The model under review builds one solid part; all positions refer to its coordinate system, in mm. A direction names the side the tool comes from. Round coordinates to 2 decimals unless told otherwise and drop trailing zeros. Write each loop counter-clockwise with the first axis right and the second up, starting at its lowest first coordinate (ties: lowest second). Pieces come first, ordered by that corner, then holes.
Item 1: Machinability: for faces 4 (the face through (-24, 38, -35)), 5 (the face through (0, 19.5, -20)), 6 (the face through (-1, 24, -80.533)), 7 (the face through (0, 22, -9.757)), which of the approach directions +Z, -Z, +X, -X, +Y, -Y give a long, thin tool a straight path to every point of the face, cutting with its end or side? Answer none if there is none.
Item 2: Add section C-C (x = 23). Give the boundary of the cut face in (y, z), plus the area to 3 significant figures.
Item 3: Add section A-A (x = -6). Give the boundary of the cut face in (y, z), plus the area to 3 significant figures.
Item 4: Draft analysis for pull direction X (two halves, no side actions). For faces 1 (the face through (23, 28, -40)), 2 (the face through (30.5, 22, -20)), 3 (the face through (0, 80, -1)), state which applies: +X half, -X half, draft (parallel to the pull), parting line (faces both ways), or undercut.
Item 5: Clearance check with flat-ended pins moving along their axes: pin 1 Ø6 at (x, y) = (-13, 41) entering from -Z; pin 2 Ø2 at (x, y) = (44, 75) entering from -Z; pin 3 Ø5 at (x, z) = (14.5, -61.5) entering from -Y; pin 4 Ø2 at (x, z) = (-25.5, -59) entering from +Y. State where each tip first meets the part, or that it passes through.
Item 6: To check wall thickness, follow L1, parallel to Z at x = -35, y = 19; L2, parallel to X at y = 59, z = -43.5; L3, parallel to Z at x = 2.5, y = 10. State the ranges of each line that lie inside material, in increasing order.
Item 7: Add section B-B (y = 11.5). Give the boundary of the cut face in (x, z), plus the area to 3 significant figures.
Item 8: Add section D-D (z = -44.5). Give the boundary of the cut face in (x, y), plus the area to 3 significant figures.
Autodesk Inventor part; units mm, degrees
ref_plane "YZ Plane" through (0, 0, 0) normal (1, 0, 0) x (0, 1, 0)
ref_plane "XZ Plane" through (0, 0, 0) normal (0, 1, 0) x (-1, 0, 0)
ref_plane "XY Plane" through (0, 0, 0) normal (0, 0, 1) x (1, 0, 0)
sketch "Esboço1" plane through (0, 0, 0) normal (1, 0, 0) x (0, 1, 0)
  line L0 (0, 0) -> (80, 0)
  line L1 (80, 0) -> (80, -52)
  line L2 (80, -97) -> (0, -97)
  line L3 (0, -97) -> (0, 0)
  line L4 (80, 0) -> (0, 0)
  line L5 (0, 0) -> (0, -60)
  line L6 (80, -60) -> (80, 0)
  line L7 (0, 0) -> (0, -19.5)
  line L8 (19.5, 0) -> (0, 0)
  line L9 (0, -98) -> (0, -97)
  line L10 (0, -97) -> (40, -97)
  line L11 (0, 0) -> (0, -20)
  line L12 (80, 0) -> (80, -52)
  line L13 (80, -52) -> (0, -52)
  line L14 (0, -52) -> (0, -97)
  line L15 (0, -97) -> (80, -97)
  line L16 (80, -97) -> (80, -52)
  line L17 (0, -74.5) -> (0, -97)
  line L18 (0, -97) -> (80, -97)
  line L19 (80, -97) -> (80, -74.5)
  line L20 (80, -52) -> (80, -78.5)
  line L21 (53.5, -78.5) -> (28.1691, -78.5)
  line L22 (80, -52) -> (53.5, -78.5)
  arc A0 (0.0257, -97) -> (0, -98) centre (19.5, -98) ccw
  line L23 (80, -52) -> (80, -54)
  line L24 (80, -54) -> (53.5, -80.533)
  line L25 (53.5, -80.533) -> (28.1691, -80.533)
  line L26 (28.1691, -80.533) -> (28.1691, -78.5)
  arc A1 (18.9926, -80.533) -> (0, -98) centre (23.5809, -104.5813) ccw
  line L27 (28.1691, -80.533) -> (18.9926, -80.533)
  circle A2 centre (20, -20) radius 18.5
  line L28 (20, -38.5) -> (0, -38.5)
  line L29 (20, -1.5) -> (0, -1.5)
  point P0 (0, -78.5)
  point P1 (80, -78.5)
  point P2 (0.3022, -97)
  dimension "d0" = 80
  dimension "d1" = 97
  dimension "d6" = 20
  dimension "d13" = 52
  dimension "d14" = 26.5
  dimension "d15" = 26.5
  dimension "d16" = 26.5
  dimension "d17" = 19.5
  dimension "d19" = 2
  dimension "d20" = 37.5
  dimension "d75" = 37
sketch "Esboço2" plane through (0, 0, 0) normal (1, 0, 0) x (0, 1, 0)
  point P0 (0, 0)
extrude "Extrusão1" add sketch "Esboço1" along normal mid plane 97 contours L0 L1 L13 L3 L28 A2 L29 | L29 A2 L28 L3 | A2 | L22 L21 L26 L27 A1 L2 L3 L13 | L2 A0 L9 | A1 A0 L2
sketch "Esboço3" plane through (0, 0, 0) normal (1, 0, 0) x (0, 1, 0)
  line L0 (0, 0) -> (80, 0)
  line L1 (80, 0) -> (80, -2.5)
  line L2 (80, 0) -> (80, -52)
  line L3 (80, -2.5) -> (80, -5)
  line L4 (80, -2.5) -> (77, -2.5)
  line L5 (53.5, -78.5) -> (28.1691, -78.5)
  line L6 (77, -2.5) -> (42, -2.5)
  line L7 (42, -2.5) -> (42, -78.5)
  line L8 (42, -78.5) -> (77, -78.5)
  line L9 (77, -78.5) -> (77, -2.5)
  line L10 (28.1691, -78.5) -> (31.1691, -78.5)
  line L11 (28.1691, -78.5) -> (42, -78.5)
  line L12 (42, -78.5) -> (42, -40.5)
  line L13 (28.1691, -78.5) -> (42, -78.5)
  line L14 (42, -78.5) -> (42, -42.2949)
  line L15 (42, -42.2949) -> (28.1691, -42.2949)
  line L16 (28.1691, -42.2949) -> (28.1691, -78.5)
  line L17 (28.1691, -42.2949) -> (4.792, -42.2949)
  line L18 (4.792, -42.2949) -> (4.792, -71.2859)
  line L19 (4.792, -71.2859) -> (28.1691, -71.2859)
  point P0 (20, 0)
  dimension "d27" = 2.5
  dimension "d28" = 2.5
  dimension "d29" = 3
  dimension "d30" = 35
extrude "Extrusão2" cut sketch "Esboço3" along normal mid plane 91
sketch "Esboço4" plane through (-48.5, 80, 0) normal (0, 1, 0) x (1, 0, 0)
  line L0 (0, 0) -> (0, 52)
  line L1 (0, 0) -> (97, 0)
  line L2 (3, 2.5) -> (3, 55)
  line L3 (94, 2.5) -> (3, 2.5)
  line L4 (3, 2.5) -> (93.6926, 2.5)
  line L5 (93.6926, 2.5) -> (93.6926, 52)
  line L6 (93.6926, 52) -> (3, 52)
  line L7 (3, 52) -> (3, 2.5)
  point P0 (48.5, 0)
extrude "Extrusão3" cut sketch "Esboço4" against normal blind 8.5
sketch "Esboço5" plane through (-45.5, 77, -52) normal (0, 0, 1) x (1, 0, 0)
  line L0 (91, 0) -> (0, 0)
  line L1 (0, 0) -> (4, 0)
  line L2 (4, 0) -> (4, -4)
  line L3 (4, -4) -> (0, -4)
  line L4 (0, -4) -> (0, 0)
  line L5 (91, -23.5) -> (91, 0)
  line L6 (91, 0) -> (87, 0)
  line L7 (87, 0) -> (87, -4)
  line L8 (87, -4) -> (91, -4)
  line L9 (91, -4) -> (91, 0)
  line L10 (0, 3) -> (0, 0)
  line L11 (0, 3) -> (4, 3)
  line L12 (4, 3) -> (4, 0)
  line L13 (4, 0) -> (0, 0)
  line L14 (0, 0) -> (0, 3)
  line L15 (87, 3) -> (91, 3)
  line L16 (91, 3) -> (91, 0)
  line L17 (91, 0) -> (87, 0)
  line L18 (87, 0) -> (87, 3)
  point P0 (45.5, -77)
  point P1 (91, -4)
  dimension "d38" = 4
  dimension "d39" = 4
  dimension "d40" = 4
extrude "Extrusão4" add sketch "Esboço5" along normal blind 49.5
sketch "Esboço6" plane through (45.5, 4.792, -42.2949) normal (0, 0, -1) x (-1, 0, 0)
  line L0 (0, 37.208) -> (0, 33.208)
  line L1 (17, 33.208) -> (27, 33.208)
  line L2 (27, 33.208) -> (27, 23.208)
  line L3 (27, 23.208) -> (17, 23.208)
  line L4 (17, 23.208) -> (17, 33.208)
  line L5 (0, 37.208) -> (91, 37.208)
  line L6 (91, 37.208) -> (87, 37.208)
  line L7 (-3, 35.208) -> (94, 35.208)
  line L8 (91, 37.208) -> (91, 33.208)
  line L9 (74, 33.208) -> (64, 33.208)
  line L10 (64, 33.208) -> (64, 23.208)
  line L11 (64, 23.208) -> (74, 23.208)
  line L12 (74, 23.208) -> (74, 33.208)
  line L13 (91, 33.208) -> (74, 33.208)
  point P0 (45.5, -4.792)
  dimension "d43" = 4
  dimension "d44" = 17
  dimension "d45" = 10
  dimension "d46" = 10
  dimension "d52" = 10
  dimension "d53" = 10
  dimension "d54" = 17
extrude "Extrusão5" cut sketch "Esboço6" against normal blind 14 contours L12 L11 L10 L9 | L1 L2 L3 L4
sketch "Esboço9" plane through (48.5, 0, 0) normal (1, 0, 0) x (0, 0, -1)
  circle A0 centre (20, 20) radius 18.5
  line L0 (1.5, 20) -> (1.5, 0)
  line L1 (98, 0) -> (0, 0)
  line L2 (38.5, 20) -> (38.5, 0)
  line L3 (20, 24) -> (1.9376, 24)
  line L4 (20, 24) -> (38.0624, 24)
  line L5 (20, 19.5) -> (38.5, 19.5)
  line L6 (20, 19.5) -> (1.5, 19.5)
  point P0 (38.5, 0)
  point P1 (1.5068, 19.5)
  point P2 (38.4932, 19.5)
  dimension "d76" = 37
  dimension "d81" = 4.5
extrude "Extrusão7" cut sketch "Esboço9" against normal blind 97
extrude "Extrusão8" add sketch "Esboço9" against normal blind 97 contours A0 L5 L6 L3 L4
sketch "Esboço10" plane through (48.5, 19.5, -38.4932) normal (0, -1, 0) x (1, 0, 0)
  line L0 (-97, 0) -> (-97, 36.9865)
  line L1 (0, -13.5068) -> (0, 38.4932)
  line L2 (0, 0.4309) -> (0, 36.5556)
  line L3 (0, -0.0068) -> (-97, -0.0068)
  line L4 (-97, 36.9865) -> (-79, 36.9865)
  line L5 (-79, 36.9865) -> (-79, -0.0068)
  line L6 (-79, -0.0068) -> (-97, -0.0068)
  line L7 (-97, -0.0068) -> (-97, 36.9865)
  line L8 (0, 36.9865) -> (-97, 36.9865)
  line L9 (-18, 36.9865) -> (0, 36.9865)
  line L10 (0, 36.9865) -> (0, -0.0068)
  line L11 (0, -0.0068) -> (-18, -0.0068)
  line L12 (-18, -0.0068) -> (-18, 36.9865)
  point P0 (-48.5, 38.4932)
extrude "Extrusão9" cut sketch "Esboço10" against normal blind 4.5 contours L0 L4 L5 L3 L7 | L8 L1 L3 L12
sketch "Esboço11" plane through (-30.5, 19.5, -1.5068) normal (0, -1, 0) x (1, 0, 0)
  line L0 (0, 0) -> (0, -36.9865)
  line L1 (0, -36.9865) -> (0, -28.7365)
  line L2 (-18, 0) -> (0, 0)
  line L3 (0, 0) -> (0, -8.25)
  line L4 (0, -28.7365) -> (0, -8.25)
  line L5 (61, 0) -> (61, -8.25)
  line L6 (61, -36.9865) -> (61, 0)
  line L7 (61, -36.9865) -> (61, -28.7365)
  line L8 (61, -28.7365) -> (61, -8.25)
  line L9 (61, -18.4932) -> (33, -18.4932)
  line L10 (33, -18.4932) -> (37, -18.4932)
  line L11 (61, -18.4932) -> (57, -18.4932)
  line L12 (37, -8.25) -> (47, -8.25)
  line L13 (47, -8.25) -> (47, -28.7365)
  line L14 (47, -28.7365) -> (37, -28.7365)
  line L15 (37, -28.7365) -> (37, -8.25)
  line L16 (38, -18.4932) -> (34, -18.4932)
  line L17 (24, -8.25) -> (14, -8.25)
  line L18 (14, -8.25) -> (14, -28.7365)
  line L19 (14, -28.7365) -> (24, -28.7365)
  line L20 (24, -28.7365) -> (24, -8.25)
  line L21 (24, -18.4932) -> (28, -18.4932)
  line L22 (24, -18.4932) -> (0, -18.4932)
  line L23 (28, -8.25) -> (33, -8.25)
  line L24 (33, -8.25) -> (33, -3.25)
  line L25 (33, -3.25) -> (28, -3.25)
  line L26 (28, -3.25) -> (28, -8.25)
  line L27 (28, -28.7365) -> (33, -28.7365)
  line L28 (33, -28.7365) -> (33, -33.7365)
  line L29 (33, -33.7365) -> (28, -33.7365)
  line L30 (28, -33.7365) -> (28, -28.7365)
  point P0 (30.5, 1.5068)
  dimension "d91" = 8.25
  dimension "d92" = 8.25
  dimension "d96" = 28
  dimension "d100" = 4
  dimension "d101" = 4
  dimension "d102" = 4
  dimension "d105" = 5
  dimension "d106" = 5
  dimension "d107" = 5
  dimension "d108" = 5
extrude "Extrusão10" cut sketch "Esboço11" against normal blind 4.5 contours L26 L25 L24 L23 | L27 L28 L29 L30
properties part number "Mini Sumô Definitivo - CHASSI"
Numbers:
1. face 4: -Z
1. face 5: +X, -X, -Y
1. face 6: -Z, +X, -X, +Y
1. face 7: -Y
2. outline: (0, -98) arc R24.48 cw to (18.99, -80.53) - (28.17, -80.53) - (28.17, -71.29) - (4.79, -71.29) - (4.79, -42.29) - (28, -42.29) - (28, -36.68) arc R18.5 cw to (24, -38.06) - (24, -1.94) arc R18.5 cw to (36.54, -28.29) - (38, -28.29) - (38, -42.29) - (42, -42.29) - (42, -2.5) - (80, -2.5) - (80, 0) - (0, 0) - (0, -1.5) - (20, -1.5) arc R18.5 ccw to (19.5, -1.51) - (19.5, -38.49) arc R18.5 ccw to (20, -38.5) - (0, -38.5) - close; (77, -55) - (80, -52) - (77, -52) - close
2. area: 1,170 mm2
3. outline: (0, -98) arc R24.48 cw to (18.99, -80.53) - (28.17, -80.53) - (28.17, -71.29) - (4.79, -71.29) - (4.79, -42.29) - (42, -42.29) - (42, -2.5) - (80, -2.5) - (80, 0) - (0, 0) - (0, -1.5) - (20, -1.5) arc R18.5 ccw to (19.5, -1.51) - (19.5, -38.49) arc R18.5 ccw to (20, -38.5) - (0, -38.5) - close; (77, -55) - (80, -52) - (77, -52) - close; hole (24, -38.06) arc R18.5 ccw to (24, -1.94) - close
3. area: 1,260 mm2
4. face 1: undercut
4. face 2: +X half
4. face 3: draft
5. pin 1: stops at z = -42.29
5. pin 2: stops at z = -52
5. pin 3: stops at y = 0
5. pin 4: stops at y = 4.79
6. L1: z = -80.53 to -71.29, -42.29 to -38.5, -1.5 to 0
6. L2: x = -48.5 to -45.5, 45.5 to 48.5
6. L3: z = -84.21 to -71.29, -42.29 to -38.5, -1.5 to 0
7. outline: (-48.5, -83.29) - (48.5, -83.29) - (48.5, -38.5) - (-48.5, -38.5) - close; (-48.5, -1.5) - (48.5, -1.5) - (48.5, 0) - (-48.5, 0) - close; hole (-45.5, -71.29) - (45.5, -71.29) - (45.5, -42.29) - (-45.5, -42.29) - close
7. area: 1,850 mm2
8. outline: (-48.5, 0) - (48.5, 0) - (48.5, 80) - (41.5, 80) - (41.5, 73) - (45.5, 73) - (45.5, 4.79) - (-45.5, 4.79) - (-45.5, 73) - (-41.5, 73) - (-41.5, 80) - (-48.5, 80) - close
8. area: 972 mm2
